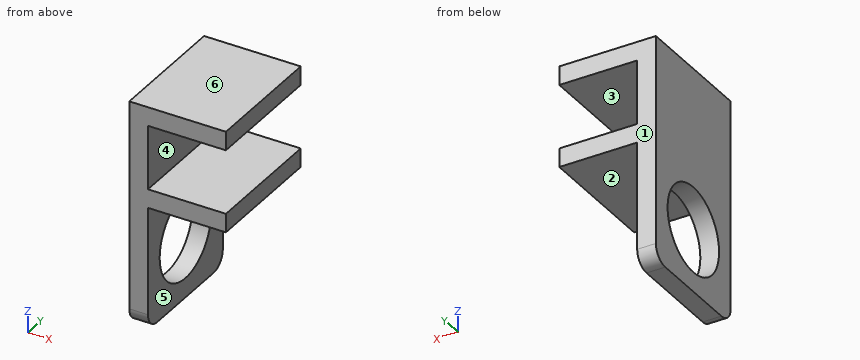
from build123d import *

# Parameters (mm, degrees)
F0_W     = 25
F0_H     = 6
F1_DEPTH = 40
F2_R     = 5
F3_R     = 13.75
F4_DEPTH = 25


with BuildPart() as f1:
    # F0 (on Front) → F1 (new body)
    with BuildSketch(Plane.XZ):
        Polygon((0, 72), (0, 0), (6, 0), (6, 39.5), (6, 45.5), (6, 66), (6, 72), align=None)
        with Locations((18.5, 42.5)):
            Rectangle(F0_W, F0_H)
        with Locations((18.5, 69)):
            Rectangle(F0_W, F0_H)
    extrude(amount=F1_DEPTH)

    # F2
    f2_edges = [f1.edges().sort_by_distance(p)[0] for p in [
        (3, 0, 0),
        (3, -40, 0),
    ]]
    fillet(f2_edges, radius=F2_R)

    # F3 (on face) → F4 (cut)
    with BuildSketch(Plane(origin=(0, 0, 0), x_dir=(0, -1, 0), z_dir=(-1, 0, 0))):
        with Locations((20, 20)):
            Circle(F3_R)
    extrude(amount=-F4_DEPTH, mode=Mode.SUBTRACT)


solid = f1.part
CAD build for the part. Positions are in the model's coordinates, mm. Face numbers are marked on the shaded views. A direction names the side the tool comes from. Coordinates: 2 decimals unless noted, no trailing zeros. Loops run counter-clockwise (first coordinate to the right, second up) from the corner with the lowest first, then second, coordinate; pieces in that order, holes last. Notation, with made-up numbers: (39, 89.5) -> (44, 89.5) arc R28 ccw to (44, 116.5) -> close; hole circle Ø1 at (50.25, 78). An arc over 180 degrees is marked (long way). One line per item, written item: value.
1. Slice it at A-A on z = 31. Write the cut outline in (x, y).
Answers:
outline: (0, -40) -> (6, -40) -> (6, -28.25) -> (0, -28.25) -> close; (0, -11.75) -> (6, -11.75) -> (6, 0) -> (0, 0) -> close
2. Slice it at D-D on x = 4. Write the cut outline in (y, z).
Answers:
outline: (-40, 5) arc R5 ccw to (-35, 0) -> (-5, 0) arc R5 ccw to (0, 5) -> (0, 72) -> (-40, 72) -> close; hole circle Ø27.5 at (-20, 20)
3. Flat gauge pins, fed straight in: P1, Ø7.5, axis at x = 16, y = -20, coming from the -Z side; P2, Ø6, axis at y = -23.5, z = 53, coming from the +X side. Where does each tip first touch, or does it go through?
Answers:
P1: stops at z = 39.5
P2: stops at x = 6
4. Slice it at C-C on y = -20. Write the cut outline in (x, z), and give its area (3 significant figures).
Answers:
outline: (0, 0) -> (6, 0) -> (6, 6.25) -> (0, 6.25) -> close; (0, 33.75) -> (6, 33.75) -> (6, 39.5) -> (31, 39.5) -> (31, 45.5) -> (6, 45.5) -> (6, 66) -> (31, 66) -> (31, 72) -> (0, 72) -> close
area: 567 mm^2
5. Pull direction Z, two halves, no side cores. Call the marked faces 1, 2 and 3: pulls with the +Z half, pulls with the -Z half, needs draft (parallel to the pull), parting line crosses it, or undercut.
Answers:
face 1: needs draft
face 2: pulls with the -Z half
face 3: undercut
6. Which spindle directions (+Z, -Z, +X, -X, +Y, -Y) get a long thin tool onto all of the face, cutting with end or side? Do the marked faces 4, 5 and 6. Say none if no direction does.
Answers:
face 4: +X, +Y, -Y
face 5: -Z, +X, +Y, -Y
face 6: +Z, +X, -X, +Y, -Y
7. Drill centre lines: line 1 (Z direction, x = 24.5, y = -18); line 2 (Z direction, x = 2.4, y = -20); line 3 (X direction, y = -36, z = 36.5). Where is each one in solid material? Low to high. Write a range as [from, to].
Answers:
line 1: z = [39.5, 45.5], [66, 72]
line 2: z = [0, 6.25], [33.75, 72]
line 3: x = [0, 6]
8. Slice it at B-B on x = 18.5. Write the cut outline in (y, z).
Answers:
outline: (-40, 39.5) -> (0, 39.5) -> (0, 45.5) -> (-40, 45.5) -> close; (-40, 66) -> (0, 66) -> (0, 72) -> (-40, 72) -> close
